Geometry check sheet. Reference: drawing and pictorial views, mm from the part's lowest x, y, z. Give positions to 0.01 mm unless a question says otherwise; leave off trailing zeros. Write each loop counter-clockwise with the first axis right and the second up, starting at its lowest first coordinate (ties: lowest second). Pieces come first, ordered by that corner, then holes. Notation, with made-up numbers: (-28.75, 15) -> (9.25, 15) arc R20 ccw to (9.25, 36) -> close; hole circle Ø1 at (-32, 40.25). An arc over 180 degrees is marked (long way). Write each question's results on one line, items separated by ' | '. Start each with the question number.
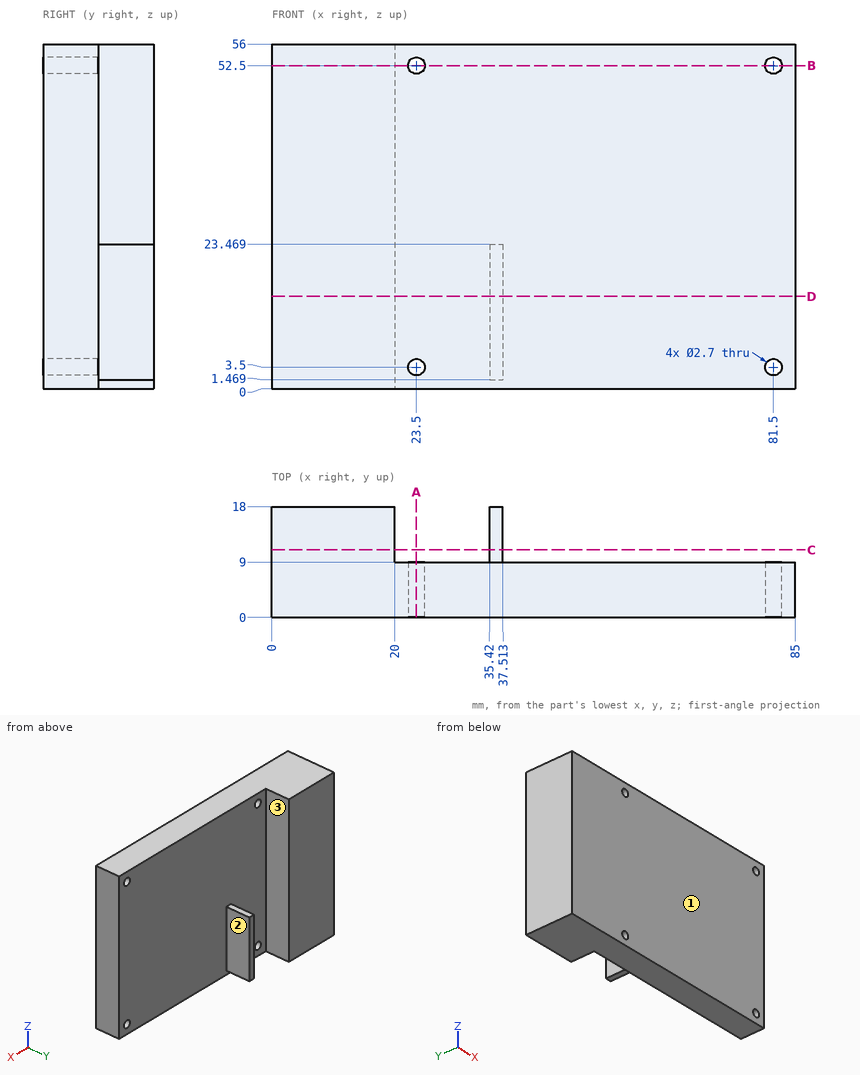
Item 1: Section check A-A on x = 23.5. Record the boundary of the cut face in (y, z).
Item 2: Thickness scan on probe 1 along X at (y, z) = (4, 3.5); probe 2 along Z at (x, y) = (23.5, 4.5); probe 3 along Y at (x, z) = (31, 24). Record the ranges inside material, lowest first. Write a range as from..to.
Item 3: Section check B-B on z = 52.5. Record the boundary of the cut face in (x, y).
Item 4: Depth check by flat-ended pin: pin 1 Ø2.5 at (y, z) = (13, 7.5) entering from +X; pin 2 Ø3.5 at (x, z) = (23.5, 52.5) entering from +Y; pin 3 Ø0.6 at (x, y) = (37, 14.5) entering from +Z. Enter the tip coordinate at first touch or a pass-through.
Item 5: Mould release check, pull along X, two halves, no side actions. Record for the marked faces 1, 2 and 3: pulls with the +X half, pulls with the -X half, needs draft (parallel to the pull), parting line crosses it, or undercut.
Item 6: Section check D-D on z = 15. Record the boundary of the cut face in (x, y).
Item 7: Section check C-C on y = 11. Record the boundary of the cut face in (x, z).
Check sheet entries:
1) outline: (0, 0) -> (9, 0) -> (9, 2.15) -> (0, 2.15) -> close; (0, 4.85) -> (9, 4.85) -> (9, 51.15) -> (0, 51.15) -> close; (0, 53.85) -> (9, 53.85) -> (9, 56) -> (0, 56) -> close
2) probe 1: x = 0..22.15, 24.85..80.15, 82.85..85 | probe 2: z = 0..2.15, 4.85..51.15, 53.85..56 | probe 3: y = 0..9
3) outline: (0, 0) -> (22.15, 0) -> (22.15, 9) -> (20, 9) -> (20, 18) -> (0, 18) -> close; (24.85, 0) -> (80.15, 0) -> (80.15, 9) -> (24.85, 9) -> close; (82.85, 0) -> (85, 0) -> (85, 9) -> (82.85, 9) -> close
4) pin 1: stops at x = 37.51 | pin 2: stops at y = 9 | pin 3: stops at z = 23.47
5) face 1: needs draft | face 2: pulls with the +X half | face 3: undercut
6) outline: (0, 0) -> (85, 0) -> (85, 9) -> (37.51, 9) -> (37.51, 18) -> (35.42, 18) -> (35.42, 9) -> (20, 9) -> (20, 18) -> (0, 18) -> close
7) outline: (0, 0) -> (20, 0) -> (20, 56) -> (0, 56) -> close; (35.42, 1.47) -> (37.51, 1.47) -> (37.51, 23.47) -> (35.42, 23.47) -> close
